Source: CAD feature listing. Evaluate the final solid. Frame: model axes, mm. A direction names the side the tool comes from. Give positions to 0.01 mm unless a question says otherwise; leave off trailing zeros. Loops run counter-clockwise (first coordinate to the right, second up) from the corner with the lowest first, then second, coordinate; pieces in that order, holes last.
Solid Edge part; units mm, degrees
sketch "Sketch1" plane through (0, 0, 0) normal (0, 0, 1) x (1, 0, 0)
  circle A0 centre (0, 0) radius 6.5
extrude "Protrusion1" add sketch "Sketch1" along normal blind 152.5
sketch "Sketch2" plane through (0, 0, 0) normal (0, 0, -1) x (1, 0, 0)
  line L0 (3.5, 5.4772) -> (3.5, -5.4772)
extrude "ExtrudedCutout_1" cut sketch "Sketch2" against normal blind 9 material side at (3.55, 0, 0)
chamfer "Chamfer_1" distance 0.75 angle 45 2 edges at (-6.5, 0, 0) (-6.5, 0, 152.5)
sketch "Sketch3" plane through (5, 0, 101) normal (0, 0, -1) x (0, 1, 0)
  circle A0 centre (0, -5) radius 8.5
extrude "ExtrudedProtrusion_2" add sketch "Sketch3" along normal blind 4
properties part number "SV-101" material "STEEL, 4140"
(1) Section A-A, the plane y = 0. Return the cut outline in (x, z).
A:
outline: (-8.5, 97) - (-6.5, 97) - (-6.5, 0.75) - (-5.75, 0) - (3.5, 0) - (3.5, 9) - (6.5, 9) - (6.5, 97) - (8.5, 97) - (8.5, 101) - (6.5, 101) - (6.5, 151.75) - (5.75, 152.5) - (-5.75, 152.5) - (-6.5, 151.75) - (-6.5, 101) - (-8.5, 101) - close
(2) Section C-C, the plane z = 87. Return the cut outline in (x, y), then the cut area to 3 significant figures.
A:
outline: circle Ø13 at (0, 0)
area: 133 mm2
(3) First-contact query: pin 1 (2 mm diameter, centred on y = -2, z = 32.5, fed in from +X); pin 2 (5 mm diameter, centred on x = -3.5, z = 111, fed in from +Y); pin 3 (2.5 mm diameter, centred on y = 2, z = 3, fed in from +X). Flat tips, straight axial feed; report the tip coordinate or a pass-through.
A:
pin 1: stops at x = 6.42
pin 2: stops at y = 6.42
pin 3: stops at x = 3.5
(4) Section B-B, the plane x = 0. Return the cut outline in (y, z).
A:
outline: (-8.5, 97) - (-6.5, 97) - (-6.5, 0.75) - (-5.75, 0) - (5.75, 0) - (6.5, 0.75) - (6.5, 97) - (8.5, 97) - (8.5, 101) - (6.5, 101) - (6.5, 151.75) - (5.75, 152.5) - (-5.75, 152.5) - (-6.5, 151.75) - (-6.5, 101) - (-8.5, 101) - close
(5) Reachability of faces 1 (the cylindrical face through (-6.494, -0.286, 48.201)), 2 (the cylindrical face through (-5.158, 3.955, 126.02)), 3 (the flat face through (5, 0, 9)) from +Z, -Z, +X, -X, +Y, -Y: full face, straight path, thin tool, end or side. Return the list, or none.
A:
face 1: -Z
face 2: +Z
face 3: -Z, +X, +Y, -Y
(6) Ray query, line 1 along Z through (x, y) = (-4.75, -6.25); line 2 along X through (y, z) = (-0.5, 71.5); line 3 along X through (y, z) = (-3, 14.5). Return the intervals inside material, ascending.
A:
line 1: z = 97 to 101
line 2: x = -6.48 to 6.48
line 3: x = -5.77 to 5.77
